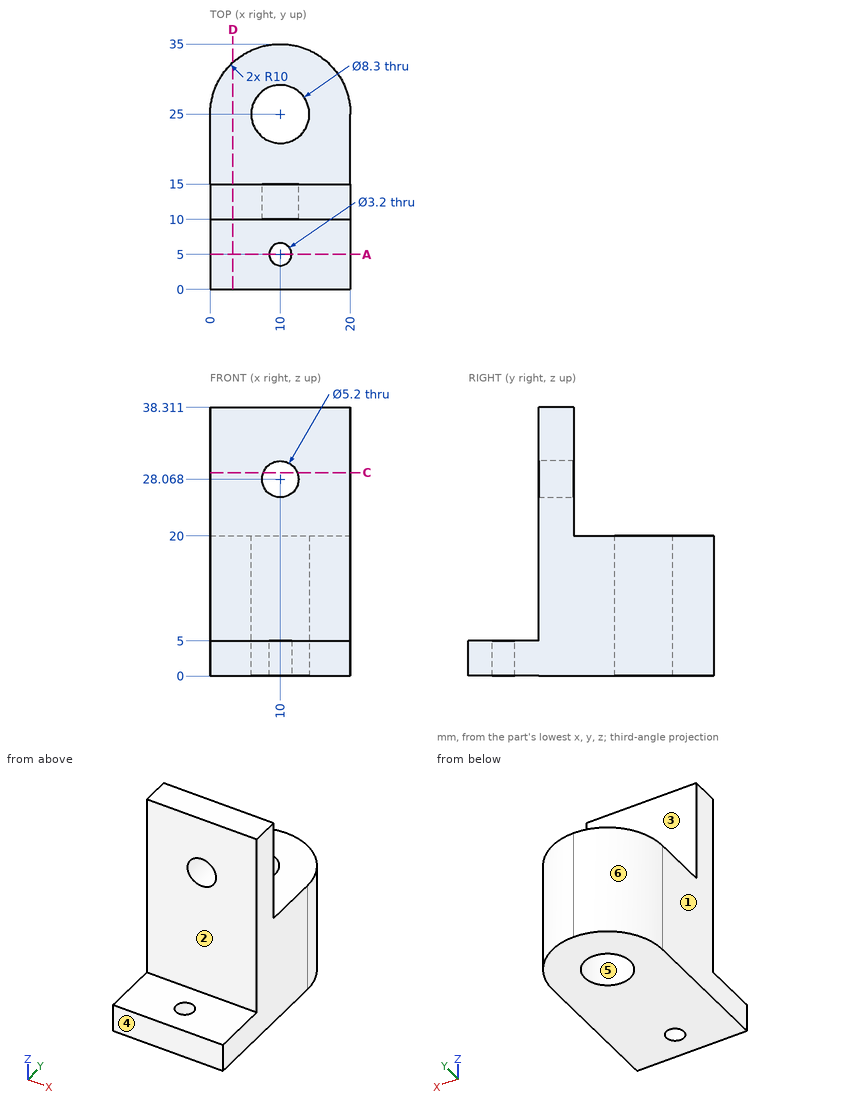
Input: dimensioned drawing with shaded views. Units: mm. Origin: part minimum x, y, z. A direction names the side the tool comes from. Give positions to 0.01 mm unless a question says otherwise; leave off trailing zeros. Write each loop counter-clockwise with the first axis right and the second up, starting at its lowest first coordinate (ties: lowest second). Pieces come first, ordered by that corner, then holes.
Q1. Section C-C, the plane z = 29. Output: boundary loops of the cut face in (x, y).
Q2. First-contact query: P1, Ø6, axis at x = 10, z = 28.07, coming from the -Y side; P2, Ø5, axis at x = 10, y = 5, coming from the +Z side; P3, Ø4, axis at x = 12.5, y = 21, coming from the +Z side. Flat tips, straight axial feed; report the tip coordinate or a pass-through.
Q3. Pull-direction query (X, two-part tool) for the marked faces 4, 5 and 6; classes: pulls with the +X half, pulls with the -X half, needs draft (parallel to the pull), parting line crosses it, or undercut.
Q4. Section A-A, the plane y = 5. Output: boundary loops of the cut face in (x, z).
Q5. Material intervals for probe 1 along Y at (x, z) = (10, 3.45); probe 2 along Y at (x, z) = (10, 14); probe 3 along Z at (x, y) = (3, 18), sorted ascending.
Q6. Set-up query: the marked faces 1, 2 and 3. Return all of +Z, -Z, +X, -X, +Y, -Y with unobstructed straight access to the full face (end or side cutting, diameter ignored); none if empty.
Q7. Section D-D, the plane x = 3.25. Output: boundary loops of the cut face in (y, z).
Filled in:
1. outline: (0, 10) - (7.57, 10) - (7.57, 15) - (0, 15) - close; (12.43, 10) - (20, 10) - (20, 15) - (12.43, 15) - close
2. P1: stops at y = 10
2. P2: stops at z = 5
2. P3: stops at z = 20
3. face 4: needs draft
3. face 5: undercut
3. face 6: pulls with the -X half
4. outline: (0, 0) - (8.4, 0) - (8.4, 5) - (0, 5) - close; (11.6, 0) - (20, 0) - (20, 5) - (11.6, 5) - close
5. probe 1: y = 0 to 3.4, 6.6 to 20.85, 29.15 to 35
5. probe 2: y = 10 to 20.85, 29.15 to 35
5. probe 3: z = 0 to 20
6. face 1: +Z, -Z, -X, +Y, -Y
6. face 2: +Z, +X, -X, -Y
6. face 3: +Z, +X, -X, +Y
7. outline: (0, 0) - (32.38, 0) - (32.38, 20) - (15, 20) - (15, 38.31) - (10, 38.31) - (10, 5) - (0, 5) - close
